from build123d import *

# Parameters (mm, degrees)
BOSS_EXTRUDE1_DEPTH = 12.7
SKETCH3_R           = 2.249999945
CUT_EXTRUDE1_DEPTH  = 1397


with BuildPart() as part:
    # Sketch1 → Boss-Extrude1 (new body)
    with BuildSketch(Plane(origin=(0, 0, 0), x_dir=(1, 0, 0), z_dir=(0, 1, 0))):
        with BuildLine():
            Line((-4.562476894, -57.790786968), (-4.562476894, -70.490786968))
            Line((-4.562476894, -70.490786968), (-10.912476894, -70.490786968))
            Line((-10.912476894, -70.490786968), (-10.912476894, -57.505177075))
            ThreePointArc((-10.912476894, -57.505177075), (-11.378381687, -55.37996522), (-12.690636511, -53.644574779))
            ThreePointArc((-12.690636511, -53.644574779), (-17.570519454, -47.321172947), (-19.50995016, -39.572800421))
            ThreePointArc((-19.50995016, -39.572800421), (-21.545440648, -19.832914743), (-22.225, 0))
            ThreePointArc((-22.225, 0), (0, 22.225), (22.225, 0))
            ThreePointArc((22.225, 0), (21.545440648, -19.832914743), (19.50995016, -39.572800421))
            ThreePointArc((19.50995016, -39.572800421), (17.570519454, -47.321172947), (12.690636511, -53.644574779))
            ThreePointArc((12.690636511, -53.644574779), (11.378381687, -55.37996522), (10.912476894, -57.505177075))
            Line((10.912476894, -57.505177075), (10.912476894, -70.490786968))
            Line((10.912476894, -70.490786968), (4.562476894, -70.490786968))
            Line((4.562476894, -70.490786968), (4.562476894, -57.790786968))
            Line((4.562476894, -57.790786968), (4.562476894, -50.400688426))
            ThreePointArc((4.562476894, -50.400688426), (5.043152587, -48.243696093), (6.394215447, -46.494898164))
            ThreePointArc((6.394215447, -46.494898164), (9.053788005, -43.052382556), (10, -38.806334656))
            ThreePointArc((10, -38.806334656), (12.024185077, -19.450074611), (12.7, 0))
            ThreePointArc((12.7, 0), (0, 12.7), (-12.7, 0))
            ThreePointArc((-12.7, 0), (-12.024185077, -19.450074611), (-10, -38.806334656))
            ThreePointArc((-10, -38.806334656), (-9.053788005, -43.052382556), (-6.394215447, -46.494898164))
            ThreePointArc((-6.394215447, -46.494898164), (-5.043152587, -48.243696093), (-4.562476894, -50.400688426))
            Line((-4.562476894, -50.400688426), (-4.562476894, -57.790786968))
        make_face()
    extrude(amount=BOSS_EXTRUDE1_DEPTH)

    # Sketch3 → Cut-Extrude1 (cut)
    with BuildSketch(Plane.ZY.offset(10.912476894)):
        with Locations((63.997982022, 6.35)):
            Circle(SKETCH3_R)
    extrude(amount=-CUT_EXTRUDE1_DEPTH, mode=Mode.SUBTRACT)


solid = part.part
The listing builds one solid part. Answer for the finished solid, in the listing's coordinates (mm). A direction names the side the tool comes from. Give positions to 0.01 mm unless a question says otherwise; leave off trailing zeros. Loops run counter-clockwise (first coordinate to the right, second up) from the corner with the lowest first, then second, coordinate; pieces in that order, holes last. Notation, with made-up numbers: M 9,61 L 18,61 A28 ccw 18,95 Z; hole C 85.5,78.5 d8. An arc over 180 degrees is marked long. Answer as CSV lines item,"result".
Item 1: The mould has two halves that part along X. Classify faces 1 (the cylindrical face through (5.03, 6.26, 48.27)), 2 (the cylindrical face through (-21.526, 6.261, 20.11)), 3 (the cylindrical face through (12.005, 6.261, 19.722)), 4 (the cylindrical face through (17.62, 6.26, 47.22)): released by +X, released by -X, zero draft, split by the parting line, or undercut.
Values follow:
face 1,"undercut"
face 2,"released by -X"
face 3,"undercut"
face 4,"released by +X"
Item 2: The part is cut by section B-B (x = 8.5). Give the vertices of the cut face in (y, z), and give its area (3 significant figures).
Values follow:
outline,"M 0,-20.54 L 12.7,-20.54 L 12.7,-9.44 L 0,-9.44 Z; M 0,44.07 L 12.7,44.07 L 12.7,70.49 L 0,70.49 Z; hole C 6.35,64 d4.5"
area,"461 mm^2"
Item 3: Which of the six approach directions +Z, -Z, +X, -X, +Y, -Y give full straight-line access (tool end or side, diameter ignored) to faces 5 (the cylindrical face through (-12.043, 6.261, 19.178)), 6 (the flat face through (10.912, 9, 64)), 7 (the flat face through (-10.912, 9, 64))?
Values follow:
face 5,"+Y, -Y"
face 6,"+Z, +X, +Y, -Y"
face 7,"+Z, -X, +Y, -Y"
Item 4: Given pin 1 Ø1 at (x, y) = (-1, 2.5) entering from -Z; pin 2 Ø12 at (x, z) = (6.5, 49) entering from -Y; pin 3 Ø3 at (y, z) = (5, 17) entering from +X; pin 4 Ø6.5 at (y, z) = (7.5, 67) entering from +X, each flat-ended and moving along its own axis, determine where each tip first touches the part or whether it passes through.
Values follow:
pin 1,"stops at z = -22.22"
pin 2,"stops at y = 0"
pin 3,"stops at x = 21.81"
pin 4,"stops at x = 10.91"
Item 5: Straight lines are drawn through the part: line 1 along X through (y, z) = (9, 3); line 2 along Z through (x, y) = (5, 5.5); line 3 along Y through (x, z) = (8, 62). For each, find the intervals that lie inside material, in ascending order. Write a range as [from, to].
Values follow:
line 1,"x = [-22.21, -12.68], [12.68, 22.21]"
line 2,"z = [-21.66, -11.67], [48.34, 61.91], [66.08, 70.49]"
line 3,"y = [0, 5.32], [7.38, 12.7]"
Item 6: The part is cut by section C-C (z = 9). Give the vertices of the cut face in (x, y), and give its area (3 significant figures).
Values follow:
outline,"M -22.09,0 L -12.56,0 L -12.56,12.7 L -22.09,12.7 Z; M 12.56,0 L 22.09,0 L 22.09,12.7 L 12.56,12.7 Z"
area,"242 mm^2"
Item 7: The part is cut by section A-A (y = 6.35). Give the vertices of the cut face in (x, z) (3 decimals).
Values follow:
outline,"M -22.225,0 A22.225 ccw 22.225,0 A289.751 ccw 19.51,39.573 A19.525 ccw 12.691,53.645 A5.08 cw 10.912,57.505 L 10.912,61.748 L 4.562,61.748 L 4.562,50.401 A5.08 ccw 6.394,46.495 A10 cw 10,38.806 A280.226 cw 12.7,0 A12.7 cw -12.7,0 A280.226 cw -10,38.806 A10 cw -6.394,46.495 A5.08 ccw -4.562,50.401 L -4.562,61.748 L -10.912,61.748 L -10.912,57.505 A5.08 cw -12.691,53.645 A19.525 ccw -19.51,39.573 A289.751 ccw Z; M -10.912,66.248 L -4.562,66.248 L -4.562,70.491 L -10.912,70.491 Z; M 4.562,66.248 L 10.912,66.248 L 10.912,70.491 L 4.562,70.491 Z"
Item 8: The part is cut by section D-D (x = 0). Give the vertices of the cut face in (y, z) (3 decimals).
Values follow:
outline,"M 0,-22.225 L 12.7,-22.225 L 12.7,-12.7 L 0,-12.7 Z"
